```python
from build123d import *

# Parameters (mm, degrees)
F0_W     = 50.8
F0_H     = 50.8
F1_DEPTH = 50.8
F2_R     = 5.08
F3_T     = -2.54


# Not quite as in the source:
# - a shell that OpenCascade refuses in one call is made with other operations: the cavity is built on its own and cut out


with BuildPart() as f1:
    # F0 (on Top) → F1 (new body)
    with BuildSketch(Plane.XY):
        Rectangle(F0_W, F0_H)
    extrude(amount=F1_DEPTH)

    # F2
    f2_edges = [f1.edges().sort_by_distance(p)[0] for p in [
        (-25.4, 0, 0),
        (-25.4, 0, 50.8),
        (-25.4, 25.4, 25.4),
        (25.4, 0, 50.8),
        (0, 25.4, 50.8),
        (0, -25.4, 50.8),
        (-25.4, -25.4, 25.4),
        (25.4, 25.4, 25.4),
        (0, 25.4, 0),
        (25.4, 0, 0),
        (25.4, -25.4, 25.4),
        (0, -25.4, 0),
    ]]
    fillet(f2_edges, radius=F2_R)

    # F3: a shell. OpenCascade refuses it in one call, so the cavity is built on its own and cut out:
    # the body offset inwards by the wall thickness, plus a prism from it out through each open face.
    f3_core = offset(f1.part, amount=F3_T, mode=Mode.PRIVATE)
    f3_exits = [f3_core.faces().sort_by_distance(p)[0] for p in [
        (0, 0, 2.54),
    ]]
    add(f3_core, mode=Mode.SUBTRACT)
    extrude(f3_exits, amount=-F3_T, mode=Mode.SUBTRACT)


solid = f1.part
```
Source: CAD feature listing. Evaluate the final solid. Frame: model axes, mm. A direction names the side the tool comes from. Give positions to 0.01 mm unless a question says otherwise; leave off trailing zeros. Write each loop counter-clockwise with the first axis right and the second up, starting at its lowest first coordinate (ties: lowest second). Pieces come first, ordered by that corner, then holes. Notation, with made-up numbers: (42, -35) - (99, -35) arc R20 cw to (99, -5) - close; hole circle Ø9 at (79.5, 72). An arc over 180 degrees is marked (long way). One line per item, written item: value. Start each with the question number.
Q1. Set-up query: faces 1 (the face through (-23.951, 23.872, 25.684)), 2 (the face through (22.136, 22.096, 25.684)), 3 (the face through (20.32, 0, 1)). Return all of +Z, -Z, +X, -X, +Y, -Y with unobstructed straight access to the full face (end or side cutting, diameter ignored); none if empty.
Q2. Material intervals for probe 1 along Y at (x, z) = (-16.5, 40); probe 2 along Z at (x, y) = (-5, 9), sorted ascending. Write a range as from..to.
Q3. Draft query along X for faces 4 (the face through (0, -25.4, 25)), 5 (the face through (-22.136, 0.284, 47.496)), 6 (the face through (23.951, 23.872, 25.684)), 7 (the face through (-23.951, -23.872, 25.684)). Return one class per face: +X half, -X half, draft (parallel to the pull), parting line (faces both ways), or undercut.
Q4. First-contact query: pin 1 Ø0.8 at (x, z) = (-4.5, 2) entering from +Y; pin 2 Ø0.8 at (y, z) = (8, 1) entering from -X; pin 3 Ø0.8 at (x, z) = (-7.5, 1) entering from -Y. Flat tips, straight axial feed; report the tip coordinate or a pass-through.
Q5. Section query D-D, the plane z = 47. Return the cut outline in (x, y), then the cut area to 3 significant figures.
Q6. Section query A-A, the plane z = 28. Return the cut outline in (x, y).
Q7. Section query B-B, the plane x = -16. Return the cut outline in (y, z), then the cut area to 3 significant figures.
Answer:
1. face 1: +Z, -Z, -X, +Y
1. face 2: none
1. face 3: -Z
2. probe 1: y = -25.4..-22.86, 22.86..25.4
2. probe 2: z = 48.26..50.8
3. face 4: draft
3. face 5: undercut
3. face 6: +X half
3. face 7: -X half
4. pin 1: stops at y = 24.64
4. pin 2: stops at x = -23.82
4. pin 3: stops at y = -23.82
5. outline: (-25.24, -20.32) arc R4.92 ccw to (-20.32, -25.24) - (20.32, -25.24) arc R4.92 ccw to (25.24, -20.32) - (25.24, 20.32) arc R4.92 ccw to (20.32, 25.24) - (-20.32, 25.24) arc R4.92 ccw to (-25.24, 20.32) - close; hole (-22.51, -20.32) arc R2.19 ccw to (-20.32, -22.51) - (20.32, -22.51) arc R2.19 ccw to (22.51, -20.32) - (22.51, 20.32) arc R2.19 ccw to (20.32, 22.51) - (-20.32, 22.51) arc R2.19 ccw to (-22.51, 20.32) - close
5. area: 503 mm2
6. outline: (-25.4, -20.32) arc R5.08 ccw to (-20.32, -25.4) - (20.32, -25.4) arc R5.08 ccw to (25.4, -20.32) - (25.4, 20.32) arc R5.08 ccw to (20.32, 25.4) - (-20.32, 25.4) arc R5.08 ccw to (-25.4, 20.32) - close; hole (-22.86, -20.32) arc R2.54 ccw to (-20.32, -22.86) - (20.32, -22.86) arc R2.54 ccw to (22.86, -20.32) - (22.86, 20.32) arc R2.54 ccw to (20.32, 22.86) - (-20.32, 22.86) arc R2.54 ccw to (-22.86, 20.32) - close
7. outline: (-25.4, 5.08) arc R5.08 ccw to (-20.32, 0) - (-20.32, 2.54) arc R2.54 cw to (-22.86, 5.08) - (-22.86, 45.72) arc R2.54 cw to (-20.32, 48.26) - (20.32, 48.26) arc R2.54 cw to (22.86, 45.72) - (22.86, 5.08) arc R2.54 cw to (20.32, 2.54) - (20.32, 0) arc R5.08 ccw to (25.4, 5.08) - (25.4, 45.72) arc R5.08 ccw to (20.32, 50.8) - (-20.32, 50.8) arc R5.08 ccw to (-25.4, 45.72) - close
7. area: 370 mm2
